Read the model definition and answer for the solid it produces. Units are mm, in the model's axes. A direction names the side the tool comes from. Coordinates: 2 decimals unless noted, no trailing zeros. Order: outer loops, then holes, each group sorted by start corner. A loop starts at its lowest first (then second) coordinate and runs counter-clockwise, first axis right, second up. Notation, with made-up numbers: (2, 73) -> (12, 73) arc R34 ccw to (12, 105) -> close; hole circle Ø9 at (38, 17). An arc over 180 degrees is marked (long way). Answer in a Markdown table with one row per item.
from build123d import *

# Parameters (mm, degrees)
SKETCH1_W           = 101.6
SKETCH1_H           = 101.6
BOSS_EXTRUDE1_DEPTH = 609.6
SKETCH2_W           = 25.4
SKETCH2_H           = 101.6
CUT_EXTRUDE1_DEPTH  = 621.093025279
FILLET1_R           = 50.8
SKETCH3_R           = 25.4
CUT_EXTRUDE2_DEPTH  = 617.440783855


with BuildPart() as part:
    # Sketch1 → Boss-Extrude1 (new body)
    with BuildSketch(Plane(origin=(0, 0, 0), x_dir=(1, 0, 0), z_dir=(0, 1, 0))):
        Rectangle(SKETCH1_W, SKETCH1_H)
    extrude(amount=BOSS_EXTRUDE1_DEPTH)

    # Sketch2 → Cut-Extrude1 (cut, through all)
    with BuildSketch(Plane.XY.offset(50.8)):
        with Locations((-38.1, 50.8)):
            Rectangle(SKETCH2_W, SKETCH2_H)
        with Locations((38.1, 50.8)):
            Rectangle(SKETCH2_W, SKETCH2_H)
    extrude(amount=-CUT_EXTRUDE1_DEPTH, mode=Mode.SUBTRACT)

    # Fillet1
    fillet1_edges = [part.edges().sort_by_distance(p)[0] for p in [
        (0, 0, -50.8),
        (0, 0, 50.8),
    ]]
    fillet(fillet1_edges, radius=FILLET1_R - 0.0001)  # a hair under: the kernel refuses the full size

    # Sketch3 → Cut-Extrude2 (cut, through all)
    with BuildSketch(Plane.ZY.offset(25.4)):
        with Locations((0, 50.8)):
            Circle(SKETCH3_R)
    extrude(amount=-CUT_EXTRUDE2_DEPTH, mode=Mode.SUBTRACT)


solid = part.part
Q1. The part is cut by section C-C (z = -34). Write down the section's boundary in (x, y), then the cut area to 3 significant figures.
Outcome:
| item | result |
|---|---|
| outline | (-50.8, 101.6) -> (-25.4, 101.6) -> (-25.4, 13.06) -> (25.4, 13.06) -> (25.4, 101.6) -> (50.8, 101.6) -> (50.8, 609.6) -> (-50.8, 609.6) -> close |
| area | 56,100 mm² |
Q2. For faces 1 (the face through (38, 101.6, 1)), 2 (the face through (-1, 326, -50.8)), 3 (the face through (-25.4, 61.4, 23.3)), determine the directions among +Z, -Z, +X, -X, +Y, -Y from which every point of the face is accessible in a straight line to the end or side of a thin tool.
Outcome:
| item | result |
|---|---|
| face 1 | +Z, -Z, +X, -Y |
| face 2 | -Z, +X, -X, +Y, -Y |
| face 3 | +Z, -Z, -X, -Y |
Q3. Consider line 1 (Y direction, x = -22, z = 1); line 2 (Z direction, x = -11, y = 50); line 3 (Y direction, x = -30, z = 23). Determine where each line is inside the solid, lowest interval first.
Outcome:
| item | result |
|---|---|
| line 1 | 0.01 to 25.42, 76.18 to 609.6 |
| line 2 | -50.79 to -25.39, 25.39 to 50.79 |
| line 3 | 101.6 to 609.6 |
Q4. For a pull along Z with two mould halves and no side action, classify faces 4 (the face through (25.4, 61.4, 23.3)), 5 (the face through (0.356, 15.276, -36.314)), 6 (the face through (-0.36, 72.22, 13.65)) as pulls with the +Z half, pulls with the -Z half, needs draft (parallel to the pull), parting line crosses it, or undercut.
Outcome:
| item | result |
|---|---|
| face 4 | needs draft |
| face 5 | pulls with the -Z half |
| face 6 | undercut |
Q5. The part is cut by section D-D (x = -30.5). Write down the section's boundary in (y, z).
Outcome:
| item | result |
|---|---|
| outline | (101.6, -50.8) -> (609.6, -50.8) -> (609.6, 50.8) -> (101.6, 50.8) -> close |
Q6. The part is cut by section B-B (z = 18). Write down the section's boundary in (x, y), then the cut area to 3 significant figures.
Outcome:
| item | result |
|---|---|
| outline | (-50.8, 101.6) -> (-25.4, 101.6) -> (-25.4, 68.72) -> (25.4, 68.72) -> (25.4, 101.6) -> (50.8, 101.6) -> (50.8, 609.6) -> (-50.8, 609.6) -> close; (-25.4, 3.3) -> (25.4, 3.3) -> (25.4, 32.88) -> (-25.4, 32.88) -> close |
| area | 54,800 mm² |
Q7. Given pin 1 (3 mm diameter, centred on x = -10, z = -17.5, fed in from -Y); pin 2 (12 mm diameter, centred on x = -1, z = 31.5, fed in from -Y); pin 3 (20.5 mm diameter, centred on x = 34, z = 23, fed in from -Y), each flat-ended and moving along its own axis, determine where each tip first touches the part or whether it passes through.
Outcome:
| item | result |
|---|---|
| pin 1 | y = 2.59 |
| pin 2 | y = 6.86 |
| pin 3 | y = 3.08 |
